from build123d import *

# Parameters (mm, degrees)
PAD003_DEPTH = 1
PAD004_DEPTH = 1
FILLET012_R  = 20
FILLET013_R  = 2
FILLET014_R  = 2
FILLET015_R  = 20
PAD005_DEPTH = 4


with BuildPart() as part:
    # Sketch008 → Pad003 (new body)
    with BuildSketch(Plane.XY.offset(94)):
        with BuildLine():
            Line((0.012651, 21), (46.627451, 21))
            ThreePointArc((46.627451, 0), (62.817867, 10.5), (46.627451, 21))
            Line((46.627451, 0), (0.012651, 0))
            Line((0.012651, 0), (0.012651, 21))
        make_face()
    extrude(amount=PAD003_DEPTH)

    # Sketch010 → Pad004 (new body)
    with BuildSketch(Plane(origin=(0, 0, 94), x_dir=(1, 0, 0), z_dir=(0, 0, -1))):
        with BuildLine():
            Line((1.500068, -19.50111), (48.401309, -19.50111))
            ThreePointArc((48.401309, -19.50111), (60.857293, -10.384488), (48.233904, -1.50111))
            Line((1.500068, -1.50111), (48.233904, -1.50111))
            Line((1.500068, -1.50111), (1.500068, -19.50111))
        make_face()
    extrude(amount=PAD004_DEPTH)

    # Fillet012
    fillet012_edges = [part.edges().sort_by_distance(p)[0] for p in [
        (46.627451, 21, 94.5),
    ]]
    fillet(fillet012_edges, radius=FILLET012_R)

    # Fillet013
    fillet013_edges = [part.edges().sort_by_distance(p)[0] for p in [
        (0.012651, 21, 94.5),
    ]]
    fillet(fillet013_edges, radius=FILLET013_R)

    # Fillet014
    fillet014_edges = [part.edges().sort_by_distance(p)[0] for p in [
        (0.012651, 0, 94.5),
    ]]
    fillet(fillet014_edges, radius=FILLET014_R)

    # Fillet015
    fillet015_edges = [part.edges().sort_by_distance(p)[0] for p in [
        (46.627451, 0, 94.5),
    ]]
    fillet(fillet015_edges, radius=FILLET015_R)

    # Sketch011 → Pad005 (new body)
    with BuildSketch(Plane(origin=(0, 0, 93), x_dir=(1, 0, 0), z_dir=(0, 0, -1))):
        with BuildLine():
            Line((35.099449, -19.488966), (48.43856, -19.488966))
            ThreePointArc((48.43856, -19.488966), (60.760017, -10.202199), (48.02877, -1.485682))
            Line((35.023422, -1.485682), (48.02877, -1.485682))
            Line((35.023422, -1.485682), (35.099449, -19.488966))
        make_face()
    extrude(amount=PAD005_DEPTH)


solid = part.part
The listing builds one solid part. Answer for the finished solid, in the listing's coordinates (mm). A direction names the side the tool comes from. Coordinates: 2 decimals unless noted, no trailing zeros. Order: outer loops, then holes, each group sorted by start corner. A loop starts at its lowest first (then second) coordinate and runs counter-clockwise, first axis right, second up. Notation, with made-up numbers: M -2.5,-11.75 L 34.5,-11.75 A26 ccw 34.5,23.25 Z; hole C 84.5,18.25 d1. An arc over 180 degrees is marked long. Use CSV: the item, a comma, the result in double quotes.
Q1. Section C-C (z = 90.05) is taken. Determine the outline of the cut face in (x, y), then the cut area to 3 significant figures.
Here are the results:
outline,"M 35.02,1.49 L 48.03,1.49 A9.5 ccw long 48.44,19.49 L 35.1,19.49 Z"
area,"435 mm2"
Q2. Given pin 1 Ø2 at (y, z) = (12.5, 90) entering from -X; pin 2 Ø11.5 at (x, y) = (19.5, 12) entering from -Z; pin 3 Ø3 at (x, z) = (43.5, 90.5) entering from -Y, each flat-ended and moving along its own axis, determine where each tip first touches the part or whether it passes through.
Here are the results:
pin 1,"x = 35.07"
pin 2,"z = 93"
pin 3,"y = 1.49"
Q3. Section A-A (x = 30.5) is taken. Determine the outline of the cut face in (y, z), then the cut area to 3 significant figures.
Here are the results:
outline,"M 0,94 L 1.5,94 L 1.5,93 L 19.5,93 L 19.5,94 L 21,94 L 21,95 L 0,95 Z"
area,"39.0 mm2"
Q4. Determine the mould class of faces 1 (the cylindrical face through (60.856, 10.637, 93.507)), 2 (the flat face through (18, 11, 93)), 3 (the flat face through (32, 11, 95)), 4 (the cylindrical face through (0.583, 0.601, 94.507)) for opening direction Z: pulls with the +Z half, pulls with the -Z half, needs draft (parallel to the pull), parting line crosses it, or undercut.
Here are the results:
face 1,"undercut"
face 2,"pulls with the -Z half"
face 3,"pulls with the +Z half"
face 4,"needs draft"
Q5. A tool of negligible diameter and unlimited length cuts with its end or side. For faces 5 (the cylindrical face through (60.762, 10.454, 91.028)), 6 (the flat face through (41, 1.486, 91)), 7 (the cylindrical face through (62.814, 10.206, 94.493)), 8 (the flat face through (42, 19.489, 91)), from which of +Z, -Z, +X, -X, +Y, -Y can it reach the whole face along a straight path? Write none if from no direction.
Here are the results:
face 5,"-Z"
face 6,"-Z, -X, -Y"
face 7,"+Z, -Z"
face 8,"-Z, -X, +Y"
Q6. Section B-B (y = 11.5) is taken. Determine the outline of the cut face in (x, z), then the cut area to 3 significant figures.
Here are the results:
outline,"M 0.01,94 L 1.5,94 L 1.5,93 L 35.07,93 L 35.07,89 L 60.7,89 L 60.7,93 L 60.8,93 L 60.8,94 L 62.77,94 L 62.77,95 L 0.01,95 Z"
area,"225 mm2"
Q7. Section D-D (x = 52.5) is taken. Determine the outline of the cut face in (y, z), then the cut area to 3 significant figures.
Here are the results:
outline,"M -0.94,94 L 1.04,94 L 1.04,93 L 1,93 L 1,89 L 19.84,89 L 19.84,93 L 19.9,93 L 19.9,94 L 21.94,94 L 21.94,95 L -0.94,95 Z"
area,"117 mm2"
Q8. Straight lines are drawn through the part: L1, parallel to Z at x = 33, y = 13.75; L2, parallel to Y at x = 44, z = 90.95; L3, parallel to Z at x = 37, y = 0.25. For each, find the intervals that lie inside material, in ascending order.
Here are the results:
L1,"93 to 95"
L2,"1.49 to 19.49"
L3,"94 to 95"
